from build123d import *

# Parameters (mm, degrees)
F1_DEPTH = 1.016


with BuildPart() as f1:
    # F0 (on Top) → F1 (new body)
    with BuildSketch(Plane.XY):
        with BuildLine():
            ThreePointArc((42.0624, 0), (-27.601786, -31.739359), (-5.83724, 41.655397))
            ThreePointArc((-5.83724, 41.655397), (-4.362841, 41.835524), (-2.883003, 41.963482))
            Line((-2.883003, 41.963482), (-2.917822, 42.470287))
            ThreePointArc((-2.917822, 42.470287), (-4.415533, 42.340784), (-5.907738, 42.158482))
            ThreePointArc((-5.907738, 42.158482), (1.91701, -42.527215), (2.090709, 42.51903))
            Line((2.090709, 42.51903), (2.115717, 43.027622))
            Line((2.115717, 43.027622), (0, 43.131654))
            Line((0, 43.131654), (0, 43.640268))
            Line((0, 43.640268), (-2.697201, 43.772892))
            Line((-2.697201, 43.772892), (-2.72215, 43.265505))
            Line((-2.72215, 43.265505), (-5.507269, 43.402453))
            Line((-5.507269, 43.402453), (-5.507269, 42.894453))
            Line((-5.507269, 42.894453), (0, 42.622334))
            Line((0, 42.622334), (0, 42.0624))
            ThreePointArc((0, 42.0624), (29.742608, 29.742608), (42.0624, 0))
        make_face()
    extrude(amount=F1_DEPTH)


solid = f1.part
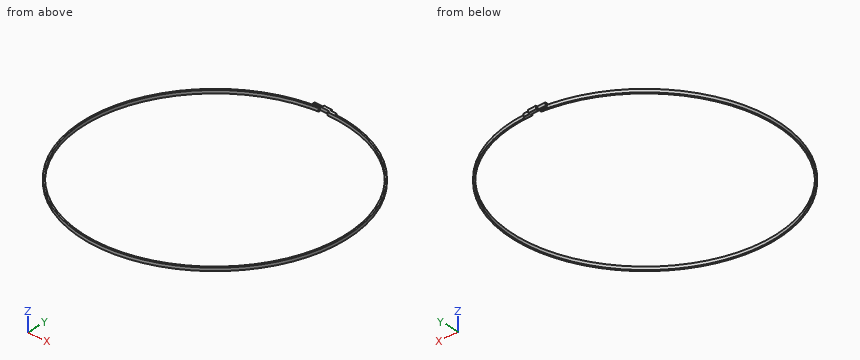
Verification items for the finished model (mm, model axes). Coordinates: 2 decimals unless noted, no trailing zeros. Order: outer loops, then holes, each group sorted by start corner. A loop starts at its lowest first (then second) coordinate and runs counter-clockwise, first axis right, second up.
Item 1: Section check C-C, the plane z = 0.2. Enter the section's corners in (x, y).
Filled in:
outline: (-5.91, 42.16) arc R42.57 ccw (long way) to (2.09, 42.52) - (2.12, 43.03) - (0, 43.13) - (0, 43.64) - (-2.7, 43.77) - (-2.72, 43.27) - (-5.51, 43.4) - (-5.51, 42.89) - (0, 42.62) - (0, 42.06) arc R42.06 cw (long way) to (-5.84, 41.66) arc R42.06 cw to (-2.88, 41.96) - (-2.92, 42.47) arc R42.57 ccw to start
Item 2: Section check A-A, the plane x = -25. Enter the section's corners in (y, z), then the cut area to 3 significant figures.
Filled in:
outline: (-34.46, 0) - (-33.83, 0) - (-33.83, 1.02) - (-34.46, 1.02) - close; (33.83, 0) - (34.46, 0) - (34.46, 1.02) - (33.83, 1.02) - close
area: 1.28 mm2
Item 3: Material ranges on L1, parallel to X at y = 36, z = 0.1; L2, parallel to X at y = -36.5, z = 0.5; L3, parallel to Y at x = 6, z = 0.55, recorded low to high.
Filled in:
L1: x = -22.72 to -21.75, 21.75 to 22.72
L2: x = -21.91 to -20.9, 20.9 to 21.91
L3: y = -42.15 to -41.63, 41.63 to 42.15
Item 4: Section check B-B, the plane y = 2. Enter the section's corners in (x, z), then the cut area to 3 significant figures.
Filled in:
outline: (-42.52, 0) - (-42.01, 0) - (-42.01, 1.02) - (-42.52, 1.02) - close; (42.01, 0) - (42.52, 0) - (42.52, 1.02) - (42.01, 1.02) - close
area: 1.03 mm2
